Input: part model. Units: mm. Frame: model coordinates. A direction names the side the tool comes from. Coordinates: 2 decimals unless noted, no trailing zeros. Order: outer loops, then holes, each group sorted by start corner. A loop starts at its lowest first (then second) coordinate and runs counter-clockwise, first axis right, second up. Notation, with made-up numbers: (-28, 87.25) -> (-21, 87.25) arc R33 cw to (-21, 122.25) -> close; hole circle Ø11 at (-5, -35). An arc over 180 degrees is marked (long way). Answer as CSV lines item,"result".
from build123d import *

# Parameters (mm, degrees)
BOSS_EXTRUDE1_DEPTH = 2


with BuildPart() as part:
    # Sketch2 → Boss-Extrude1 (new body)
    with BuildSketch(Plane.XY):
        with BuildLine():
            Line((2.381551342, -4.687082444), (1.359756513, -2.917281885))
            ThreePointArc((1.359756513, -2.917281885), (1.227533074, -2.806917507), (1.055307842, -2.808260202))
            ThreePointArc((1.055307842, -2.808260202), (0, -3), (-1.055307842, -2.808260202))
            ThreePointArc((-1.055307842, -2.808260202), (-1.227533074, -2.806917507), (-1.359756513, -2.917281885))
            Line((-1.359756513, -2.917281885), (-2.381551342, -4.687082444))
            ThreePointArc((-2.381551342, -4.687082444), (-2.532638949, -4.803371457), (-2.721774726, -4.779324465))
            ThreePointArc((-2.721774726, -4.779324465), (-4.763139721, -2.75), (-5.499903763, 0.032536177))
            ThreePointArc((-5.499903763, 0.032536177), (-5.426161181, 0.20835606), (-5.249908137, 0.28105726))
            Line((-5.249908137, 0.28105726), (-3.206318479, 0.28105726))
            ThreePointArc((-3.206318479, 0.28105726), (-3.044628404, 0.340383927), (-2.959678596, 0.490206701))
            ThreePointArc((-2.959678596, 0.490206701), (-2.64255111, 1.420184366), (-2.041957666, 2.197819122))
            ThreePointArc((-2.041957666, 2.197819122), (-1.88784416, 2.489763038), (-1.949271241, 2.814122309))
            Line((-1.949271241, 2.814122309), (-2.98980978, 4.616387925))
            Line((-2.98980978, 4.616387925), (-3.684292593, 5.819267442))
            ThreePointArc((-3.684292593, 5.819267442), (-4.381355766, 6.304889969), (-5.200363425, 6.079162791))
            ThreePointArc((-5.200363425, 6.079162791), (0, -8), (5.200363425, 6.079162791))
            ThreePointArc((5.200363425, 6.079162791), (4.381355766, 6.304889969), (3.684292593, 5.819267442))
            Line((3.684292593, 5.819267442), (2.98980978, 4.616387925))
            Line((2.98980978, 4.616387925), (1.949271241, 2.814122309))
            ThreePointArc((1.949271241, 2.814122309), (1.88784416, 2.489763038), (2.041957666, 2.197819122))
            ThreePointArc((2.041957666, 2.197819122), (2.64255111, 1.420184366), (2.959678596, 0.490206701))
            ThreePointArc((2.959678596, 0.490206701), (3.044628404, 0.340383927), (3.206318479, 0.28105726))
            Line((3.206318479, 0.28105726), (5.249908137, 0.28105726))
            ThreePointArc((5.249908137, 0.28105726), (5.426161181, 0.20835606), (5.499903763, 0.032536177))
            ThreePointArc((5.499903763, 0.032536177), (4.763139721, -2.75), (2.721774726, -4.779324465))
            ThreePointArc((2.721774726, -4.779324465), (2.532638949, -4.803371457), (2.381551342, -4.687082444))
        make_face()
    extrude(amount=BOSS_EXTRUDE1_DEPTH)


solid = part.part
1. Mould query, pull axis X, two halves, no side actions, for faces 1 (the face through (0, -4, 0)), 2 (the face through (4.393, 6.307, 0.986)), 3 (the face through (0, -8, 1)). Classes: released by +X, released by -X, zero draft, split by the parting line, or undercut.
Findings:
face 1,"zero draft"
face 2,"undercut"
face 3,"split by the parting line"
2. Ray query, line 1 along X through (y, z) = (1, 1.1); line 2 along Y through (x, z) = (-2.5, 1.75); line 3 along X through (y, z) = (-4.75, 0.2). Return the intervals inside material, ascending.
Findings:
line 1,"x = -7.94 to -2.83, 2.83 to 7.94"
line 2,"y = -7.6 to -4.79, 1.66 to 3.77"
line 3,"x = -6.44 to -2.77, -2.43 to 2.43, 2.77 to 6.44"
3. Cut plane D-D (x = 0). Return the cut outline in (y, z), plus the area to 4 significant figures.
Findings:
outline,"(-8, 0) -> (-3, 0) -> (-3, 2) -> (-8, 2) -> close"
area,"10.00 mm2"
4. Contact query for a flat-ended pin moving along its axis: pin 1 (1 mm diameter, centred on x = -4.5, z = 0.5, fed in from -Y). Output: stop coordinate, or through.
Findings:
pin 1,"stops at y = -6.93"
5. Reachability of faces 4 (the face through (-2.65, 1.41, 0.99)), 5 (the face through (0, -4, 2)) from +Z, -Z, +X, -X, +Y, -Y: full face, straight path, thin tool, end or side. Return the list, or none.
Findings:
face 4,"+Z, -Z"
face 5,"+Z, +X, -X, +Y, -Y"
6. Cut plane A-A (y = 4). Return the cut outline in (x, z).
Findings:
outline,"(-6.93, 0) -> (-2.63, 0) -> (-2.63, 2) -> (-6.93, 2) -> close; (2.63, 0) -> (6.93, 0) -> (6.93, 2) -> (2.63, 2) -> close"
7. Cut plane B-B (x = -4). Return the cut outline in (y, z), plus the area to 3 significant figures.
Findings:
outline,"(-6.93, 0) -> (-3.77, 0) -> (-3.77, 2) -> (-6.93, 2) -> close; (0.28, 0) -> (6.15, 0) -> (6.15, 2) -> (0.28, 2) -> close"
area,"18.1 mm2"
8. Cut plane C-C (z = 0.3). Return the cut outline in (x, y).
Findings:
outline,"(-5.5, 0.03) arc R0.25 cw to (-5.25, 0.28) -> (-3.21, 0.28) arc R0.25 ccw to (-2.96, 0.49) arc R3 cw to (-2.04, 2.2) arc R0.5 ccw to (-1.95, 2.81) -> (-3.68, 5.82) arc R1 ccw to (-5.2, 6.08) arc R8 ccw (long way) to (5.2, 6.08) arc R1 ccw to (3.68, 5.82) -> (1.95, 2.81) arc R0.5 ccw to (2.04, 2.2) arc R3 cw to (2.96, 0.49) arc R0.25 ccw to (3.21, 0.28) -> (5.25, 0.28) arc R0.25 cw to (5.5, 0.03) arc R5.5 cw to (2.72, -4.78) arc R0.25 cw to (2.38, -4.69) -> (1.36, -2.92) arc R0.25 ccw to (1.06, -2.81) arc R3 cw to (-1.06, -2.81) arc R0.25 ccw to (-1.36, -2.92) -> (-2.38, -4.69) arc R0.25 cw to (-2.72, -4.78) arc R5.5 cw to start"
